Check sheet for the modelled part. Datum: model origin and axes. Units: mm. Face numbers are marked on the shaded views. A direction names the side the tool comes from. Give positions to 0.01 mm unless a question says otherwise; leave off trailing zeros. Write each loop counter-clockwise with the first axis right and the second up, starting at its lowest first coordinate (ties: lowest second). Pieces come first, ordered by that corner, then holes. Notation, with made-up numbers: (78.25, 79) -> (99.25, 79) arc R36 ccw to (99.25, 115) -> close; hole circle Ø1 at (-0.5, -20.75). An arc over 180 degrees is marked (long way). Return JSON: item names as keys, results as strings.
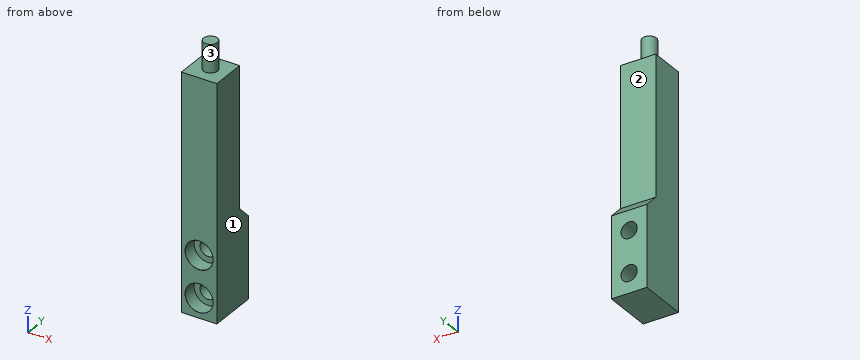
from build123d import *

# Parameters (mm, degrees)
SKETCH2_W                     = 12.7
SKETCH2_H                     = 84
BOSS_EXTRUDE1_DEPTH           = 12.7
SKETCH5_W                     = 12.7
SKETCH5_H                     = 29
BOSS_EXTRUDE2_DEPTH           = 5
CBORE_FOR_M5_SHCS1_AT_2_COUNT = 2
CBORE_FOR_M5_SHCS1_AT_2_PITCH = 15
CHAMFER1_SIZE                 = 5
SKETCH6_R                     = 2.5
BOSS_EXTRUDE3_DEPTH           = 10


with BuildPart() as part:
    # Sketch2 → Boss-Extrude1 (new body)
    with BuildSketch(Plane(origin=(0, 0, 0), x_dir=(1, 0, 0), z_dir=(0, 1, 0))):
        Rectangle(SKETCH2_W, SKETCH2_H)
    extrude(amount=BOSS_EXTRUDE1_DEPTH)

    # Sketch5 → Boss-Extrude2 (add)
    with BuildSketch(Plane(origin=(0, 12.7, 0), x_dir=(1, 0, 0), z_dir=(0, 1, 0))):
        with Locations((0, 27.5)):
            Rectangle(SKETCH5_W, SKETCH5_H)
    extrude(amount=BOSS_EXTRUDE2_DEPTH)

    # Sketch4 → CBORE for M5 SHCS1 (revolve, cut)
    with BuildSketch(Plane(origin=(0, 0, -35), x_dir=(0, 0, -1), z_dir=(1, 0, 0))):
        Polygon((0, 0), (0, 17.7), (2.9, 17.7), (2.9, 5), (5, 5), (5, 0.020977491), (5.025, 0), align=None)
    cbore_for_m5_shcs1 = revolve(axis=Axis((0, -6.35, -35), (0, 1, 0)), mode=Mode.SUBTRACT)

    # CBORE for M5 SHCS1 at 2: CBORE for M5 SHCS1 ×2
    with Locations(*[(0, 0, i * CBORE_FOR_M5_SHCS1_AT_2_PITCH) for i in range(1, CBORE_FOR_M5_SHCS1_AT_2_COUNT)]):
        add(cbore_for_m5_shcs1, mode=Mode.SUBTRACT)

    # Chamfer1
    chamfer1_edges = [part.edges().sort_by_distance(p)[0] for p in [
        (0, 12.7, -13),
    ]]
    chamfer(chamfer1_edges, length=CHAMFER1_SIZE - 0.0001)  # a hair under: the kernel refuses the full size

    # Sketch6 → Boss-Extrude3 (add)
    with BuildSketch(Plane.XY.offset(42)):
        with Locations((0, 6.35)):
            Circle(SKETCH6_R)
    extrude(amount=BOSS_EXTRUDE3_DEPTH)


solid = part.part
(1) Depth check by flat-ended pin: pin 1 Ø2 at (x, z) = (-3.5, 36.5) entering from +Y; pin 2 Ø3 at (x, z) = (1, -35) entering from -Y; pin 3 Ø2 at (x, y) = (-0.5, 10.5) entering from +Z. Enter the tip coordinate at first touch or a pass-through.
Reply:
{"pin 1": "y = 12.7", "pin 2": "through", "pin 3": "z = 42"}
(2) Cross-section at C-C on z = -35. Enter the section's corners in (x, y) (3 decimals).
Reply:
{"outline": "(-6.35, 0) -> (-5.025, 0) -> (-5, 0.021) -> (-5, 5) -> (-2.9, 5) -> (-2.9, 17.7) -> (-6.35, 17.7) -> close; (2.9, 5) -> (5, 5) -> (5, 0.021) -> (5.025, 0) -> (6.35, 0) -> (6.35, 17.7) -> (2.9, 17.7) -> close"}
(3) Thickness scan on L1, parallel to Z at x = 0, y = 8; L2, parallel to X at y = 9.25, z = -20; L3, parallel to X at y = 3, z = -35. Record the ranges inside material, lowest first.
Reply:
{"L1": "-42 to -37.9, -32.1 to -22.9, -17.1 to 52", "L2": "-6.35 to -2.9, 2.9 to 6.35", "L3": "-6.35 to -5, 5 to 6.35"}
(4) Set-up check for the marked faces 1, 2 and 3: record each of +Z, -Z, +X, -X, +Y, -Y from which the full face is reachable in a straight line by a thin tool's end or side.
Reply:
{"face 1": "+Z, -Z, +X, +Y, -Y", "face 2": "+Z, +X, -X, +Y", "face 3": "+Z"}
(5) Cross-section at A-A on x = 0. State how many separate pieces and enclosed holes the cut face has, then the cut area to 3 significant figures.
Reply:
{"separate pieces": "3", "enclosed holes": "0", "area": "1,030 mm^2"}
(6) Cross-section at B-B on y = 2.75. Enter the section's corners in (x, z).
Reply:
{"outline": "(-6.35, -42) -> (6.35, -42) -> (6.35, 42) -> (-6.35, 42) -> close; hole circle Ø10 at (0, -35); hole circle Ø10 at (0, -20)"}
(7) Cross-section at D-D on y = 6.35. Enter the section's corners in (x, z).
Reply:
{"outline": "(-6.35, -42) -> (6.35, -42) -> (6.35, 42) -> (2.5, 42) -> (2.5, 52) -> (-2.5, 52) -> (-2.5, 42) -> (-6.35, 42) -> close; hole circle Ø5.8 at (0, -35); hole circle Ø5.8 at (0, -20)"}
